Read the model definition and answer for the solid it produces. Units are mm, in the model's axes. Face numbers are marked on the shaded views. A direction names the side the tool comes from. Round coordinates to 2 decimals unless told otherwise and drop trailing zeros. Write each loop counter-clockwise with the first axis right and the second up, starting at its lowest first coordinate (ties: lowest second). Pieces come first, ordered by that corner, then holes. Notation, with made-up numbers: (16, -25.5) -> (20, -25.5) arc R16 ccw to (20, -20.5) -> close; hole circle Ø5 at (60.25, 38). An arc over 180 degrees is marked (long way). Return JSON: item names as keys, results as strings. Group by question number.
(1) Given pin 1 (9 mm diameter, centred on x = 0, y = 15, fed in from -Z); pin 2 (5 mm diameter, centred on x = -6, y = 17.5, fed in from -Z); pin 3 (6.5 mm diameter, centred on x = -13.5, y = 28.5, fed in from -Z); pin 4 (1.6 mm diameter, centred on y = 16, z = -1, fed in from -X), each flat-ended and moving along its own axis, determine where each tip first touches the part or whether it passes through.
(2) The mould has two halves that part along Z. Classify the marked faces 1, 2 and 3: released by +Z, released by -Z, zero draft, split by the parting line, or undercut.
(3) A cutting plane is placed at A-A on x = -4. Give the vertices of the cut face in (y, z), then the cut area to 3 significant figures.
(4) For the marked faces 4 and 5, determine the directions among +Z, -Z, +X, -X, +Y, -Y from which every point of the face is accessible in a straight line to the end or side of a thin tool.
(5) A cutting plane is placed at D-D on x = 0. Give the vertices of the cut face in (y, z), then the cut area to 3 significant figures.
(6) Straight lines are drawn through the part: line 1 (X direction, y = 29.5, z = -1.25); line 2 (Z direction, x = -5.25, y = 3); line 3 (Z direction, x = -4.25, y = 17.5). For each, find the intervals that lie inside material, in ascending order.
(7) A cutting plane is placed at B-B on y = 8. Give the vertices of the cut face in (x, z), then the cut area to 3 significant figures.
(8) A cutting plane is placed at C-C on z = -0.5. Give the vertices of the cut face in (x, y).
Autodesk Inventor part; units mm, degrees
ref_plane "YZ Plane" through (0, 0, 0) normal (1, 0, 0) x (0, 1, 0)
ref_plane "XZ Plane" through (0, 0, 0) normal (0, 1, 0) x (-1, 0, 0)
ref_plane "XY Plane" through (0, 0, 0) normal (0, 0, 1) x (1, 0, 0)
sketch "Szkic1" plane through (0, 0, 0) normal (0, 1, 0) x (-1, 0, 0)
  arc A0 (11.3, 0) -> (10.5, -0.8) centre (11.3, -0.8) ccw
  line L0 (10.5, -0.8) -> (10.5, -1.5)
  arc A1 (10.5, -1.5) -> (10.8, -1.8) centre (10.8, -1.5) ccw
  line L1 (10.8, -1.8) -> (12.9176, -1.8)
  arc A2 (13.5062, -3.221) -> (12.9176, -1.8) centre (12.9176, -2.6324) ccw
  line L2 (13.5062, -3.221) -> (11.2559, -5.4713)
  arc A3 (9.1346, -6.35) -> (11.2559, -5.4713) centre (9.1346, -3.35) ccw
  line L3 (9.1346, -6.35) -> (6.8654, -6.35)
  arc A4 (4.7441, -5.4713) -> (6.8654, -6.35) centre (6.8654, -3.35) ccw
  line L4 (4.7441, -5.4713) -> (2.4938, -3.221)
  arc A5 (3.0824, -1.8) -> (2.4938, -3.221) centre (3.0824, -2.6324) ccw
  line L5 (3.0824, -1.8) -> (5.2, -1.8)
  arc A6 (5.2, -1.8) -> (5.5, -1.5) centre (5.2, -1.5) ccw
  line L6 (5.5, -1.5) -> (5.5, -0.8)
  arc A7 (5.5, -0.8) -> (4.7, 0) centre (4.7, -0.8) ccw
  line L7 (0, 0) -> (4.7, 0)
  arc A8 (0, 0) -> (-2, -2) centre (0, -2) ccw
  line L8 (-2, -6.7) -> (-2, -2)
  arc A9 (-2, -6.7) -> (-1.2, -7.5) centre (-1.2, -6.7) ccw
  line L9 (-1.2, -7.5) -> (-0.5, -7.5)
  arc A10 (-0.5, -7.5) -> (-0.2, -7.2) centre (-0.5, -7.2) ccw
  line L10 (-0.2, -7.2) -> (-0.2, -5.0824)
  arc A11 (1.221, -4.4938) -> (-0.2, -5.0824) centre (0.6324, -5.0824) ccw
  line L11 (1.221, -4.4938) -> (3.4713, -6.7441)
  arc A12 (4.35, -8.8654) -> (3.4713, -6.7441) centre (1.35, -8.8654) ccw
  line L12 (4.35, -8.8654) -> (4.35, -11.1346)
  arc A13 (3.4713, -13.2559) -> (4.35, -11.1346) centre (1.35, -11.1346) ccw
  line L13 (3.4713, -13.2559) -> (1.221, -15.5062)
  arc A14 (-0.2, -14.9176) -> (1.221, -15.5062) centre (0.6324, -14.9176) ccw
  line L14 (-0.2, -14.9176) -> (-0.2, -12.8)
  arc A15 (-0.2, -12.8) -> (-0.5, -12.5) centre (-0.5, -12.8) ccw
  line L15 (-0.5, -12.5) -> (-1.2, -12.5)
  arc A16 (-1.2, -12.5) -> (-2, -13.3) centre (-1.2, -13.3) ccw
  line L16 (-2, -18) -> (-2, -13.3)
  arc A17 (-2, -18) -> (0, -20) centre (0, -18) ccw
  line L17 (4.7, -20) -> (0, -20)
  arc A18 (4.7, -20) -> (5.5, -19.2) centre (4.7, -19.2) ccw
  line L18 (5.5, -19.2) -> (5.5, -18.5)
  arc A19 (5.5, -18.5) -> (5.2, -18.2) centre (5.2, -18.5) ccw
  line L19 (5.2, -18.2) -> (3.0824, -18.2)
  arc A20 (2.4938, -16.779) -> (3.0824, -18.2) centre (3.0824, -17.3676) ccw
  line L20 (2.4938, -16.779) -> (4.7441, -14.5287)
  arc A21 (6.8654, -13.65) -> (4.7441, -14.5287) centre (6.8654, -16.65) ccw
  line L21 (6.8654, -13.65) -> (9.1346, -13.65)
  arc A22 (11.2559, -14.5287) -> (9.1346, -13.65) centre (9.1346, -16.65) ccw
  line L22 (11.2559, -14.5287) -> (13.5062, -16.779)
  arc A23 (12.9176, -18.2) -> (13.5062, -16.779) centre (12.9176, -17.3676) ccw
  line L23 (12.9176, -18.2) -> (10.8, -18.2)
  arc A24 (10.8, -18.2) -> (10.5, -18.5) centre (10.8, -18.5) ccw
  line L24 (10.5, -18.5) -> (10.5, -19.2)
  arc A25 (10.5, -19.2) -> (11.3, -20) centre (11.3, -19.2) ccw
  line L25 (16, -20) -> (11.3, -20)
  arc A26 (16, -20) -> (18, -18) centre (16, -18) ccw
  line L26 (18, -13.3) -> (18, -18)
  arc A27 (18, -13.3) -> (17.2, -12.5) centre (17.2, -13.3) ccw
  line L27 (17.2, -12.5) -> (16.5, -12.5)
  arc A28 (16.5, -12.5) -> (16.2, -12.8) centre (16.5, -12.8) ccw
  line L28 (16.2, -12.8) -> (16.2, -14.9176)
  arc A29 (14.779, -15.5062) -> (16.2, -14.9176) centre (15.3676, -14.9176) ccw
  line L29 (14.779, -15.5062) -> (12.5287, -13.2559)
  arc A30 (11.65, -11.1346) -> (12.5287, -13.2559) centre (14.65, -11.1346) ccw
  line L30 (11.65, -11.1346) -> (11.65, -8.8654)
  arc A31 (12.5287, -6.7441) -> (11.65, -8.8654) centre (14.65, -8.8654) ccw
  line L31 (12.5287, -6.7441) -> (14.779, -4.4938)
  arc A32 (16.2, -5.0824) -> (14.779, -4.4938) centre (15.3676, -5.0824) ccw
  line L32 (16.2, -5.0824) -> (16.2, -7.2)
  arc A33 (16.2, -7.2) -> (16.5, -7.5) centre (16.5, -7.2) ccw
  line L33 (16.5, -7.5) -> (17.2, -7.5)
  arc A34 (17.2, -7.5) -> (18, -6.7) centre (17.2, -6.7) ccw
  line L34 (18, -2) -> (18, -6.7)
  arc A35 (18, -2) -> (16, 0) centre (16, -2) ccw
  line L35 (11.3, 0) -> (16, 0)
  circle A36 centre (8, -10) radius 2.15
  line L36 (18, 2) -> (-2, 2)
  line L37 (-2, 2) -> (-2, 0)
  line L38 (-2, 0) -> (18, 0)
  line L39 (18, 0) -> (18, 2)
  line L40 (10.5, -1.8) -> (5.5, -1.8)
  line L41 (5.5, -1.8) -> (5.5, 0)
  line L42 (5.5, 0) -> (10.5, 0)
  line L43 (10.5, 0) -> (10.5, -1.8)
  point P0 (0, 0)
  point P1 (16, 0)
  point P2 (4.7, 0)
  dimension "d0" = 2
extrude "Wyciągnięcie proste1" add sketch "Szkic1" along normal blind 50 contours L38 L7 L37 L36 L39 L35 | L0 L43 L40 L41 L6 L38 | A1 L1 A2 L2 A3 L3 A4 L4 A5 L5 A6 L41 L40 L43
thicken "Pogrubienie1" operation add thickness 0.5 both sides no extend neighbours yes toward (-1, 0, 0) faces at (-5.5, 16.6667, -1.0333) (-5.4479, 33.3333, -1.669) (-4.4941, 16.6667, -1.8) (-2.4938, 33.3333, -2.0438) (-3.2439, 16.6667, -3.9711) (-5.5386, 33.3333, -6.0406) (-7.6218, 16.6667, -6.35) (-10.6346, 33.3333, -5.9481) (-12.006, 16.6667, -4.7212) (-13.1748, 33.3333, -1.8407) (-12.2117, 16.6667, -1.8) (-10.5402, 33.3333, -1.65) (-10.5, 16.6667, -1.2667)
properties part number "ZItemSpacer"
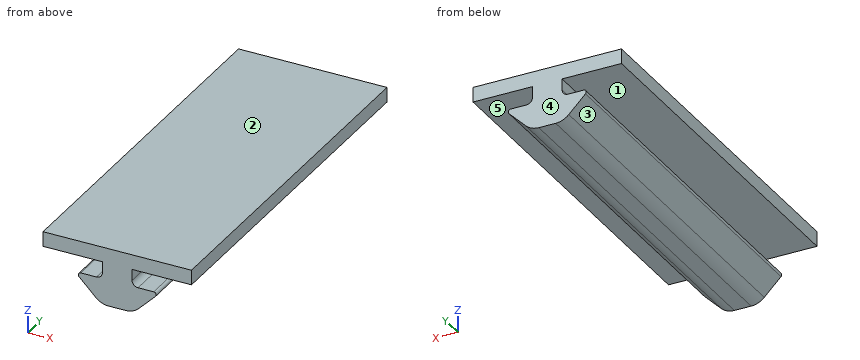
Checks:
{
 "1": {"pin 1": "stops at z = -4.52", "pin 2": "stops at z = -5.85", "pin 3": "stops at z = -5.59", "pin 4": "stops at x = -10.06"},
 "2": {"face 1": "undercut", "face 2": "released by +Z", "face 3": "released by -Z"},
 "3": {"outline": "(0, -4.02) -> (50, -4.02) -> (50, -2.3) -> (0, -2.3) -> close; (0, 0) -> (50, 0) -> (50, 2) -> (0, 2) -> close", "area": "186 mm^2"},
 "4": {"face 4": "+Z, -Z, +X, -X, +Y", "face 5": "+X, +Y, -Y"},
 "5": {"outline": "(0, 0) -> (50, 0) -> (50, 2) -> (0, 2) -> close", "area": "100 mm^2"},
 "6": {"line 1": "x = -10 to -6", "line 2": "z = -5.26 to -2.3, 0 to 2", "line 3": "z = -4.27 to -2.3, 0 to 2"},
 "7": {"outline": "(-18, 0) -> (-10, 0) -> (-10, -1.5) arc R0.8 cw to (-10.8, -2.3) -> (-12.92, -2.3) arc R0.33 ccw to (-13.15, -2.87) -> (-10.9, -5.12) arc R2.5 ccw to (-9.13, -5.85) -> (-6.87, -5.85) arc R2.5 ccw to (-5.1, -5.12) -> (-2.85, -2.87) arc R0.33 ccw to (-3.08, -2.3) -> (-5.2, -2.3) arc R0.8 cw to (-6, -1.5) -> (-6, 0) -> (2, 0) -> (2, 2) -> (-18, 2) -> close", "area": "76.9 mm^2"},
 "8": {"outline": "(-10, 0) -> (-6, 0) -> (-6, 50) -> (-10, 50) -> close"}
}
